The model under review builds one solid part; all positions refer to its coordinate system, in mm. A direction names the side the tool comes from. Coordinates: 2 decimals unless noted, no trailing zeros. Loops run counter-clockwise (first coordinate to the right, second up) from the corner with the lowest first, then second, coordinate; pieces in that order, holes last. Notation, with made-up numbers: M 17.5,80.5 L 45.5,80.5 A21 cw 45.5,86.5 Z; hole C -15,19 d2. An arc over 180 degrees is marked long. One line per item, written item: value.
```python
from build123d import *

# Parameters (mm, degrees)
SKETCH1_R               = 41.275
BOSS_EXTRUDE1_DEPTH     = 6.35
CUT_EXTRUDE1_DEPTH      = 60.737268518
CUT_EXTRUDE1_DEPTH_BACK = 60.737268518
SKETCH2_R               = 12.500000019
SKETCH3_R               = 16.000000004
CUT_EXTRUDE2_DEPTH      = 5


with BuildPart() as part:
    # Sketch1 → Boss-Extrude1 (new, symmetric)
    with BuildSketch(Plane.XY):
        Circle(SKETCH1_R)
    extrude(amount=BOSS_EXTRUDE1_DEPTH, both=True)

    # Sketch2 → Cut-Extrude1 (cut, two sides: drawn at the far end of the back side and taken through both)
    with BuildSketch(Plane.XY.offset(6.35).offset(-CUT_EXTRUDE1_DEPTH_BACK)):
        Circle(SKETCH2_R)
    extrude(amount=CUT_EXTRUDE1_DEPTH + CUT_EXTRUDE1_DEPTH_BACK, mode=Mode.SUBTRACT)

    # Sketch3 → Cut-Extrude2 (cut)
    with BuildSketch(Plane.XY.offset(6.35)):
        Circle(SKETCH3_R)
    extrude(amount=-CUT_EXTRUDE2_DEPTH, mode=Mode.SUBTRACT)


solid = part.part
```
(1) Add section A-A on x = 0. State the section outline as (y, z) points (3 decimals).
Checks:
outline: M -41.275,-6.35 L -12.5,-6.35 L -12.5,1.35 L -16,1.35 L -16,6.35 L -41.275,6.35 Z; M 12.5,-6.35 L 41.275,-6.35 L 41.275,6.35 L 16,6.35 L 16,1.35 L 12.5,1.35 Z
(2) Insertion check: pin 1 Ø1.5 at (y, z) = (12.5, -1.5) entering from +X; pin 2 Ø3 at (y, z) = (-20, 3) entering from +X; pin 3 Ø6 at (y, z) = (-27, -1) entering from +X. Each pin has a flat end and moves straight along its axis. Give the tip position at first contact, or say it passes through.
Checks:
pin 1: x = 39.57
pin 2: x = 36.9
pin 3: x = 33.58
(3) Add section C-C on z = -2.25. State the section outline as (x, y) points (3 decimals), then the cut area to 3 significant figures.
Checks:
outline: C 0,0 d82.55; hole C 0,0 d25
area: 4,860 mm^2
(4) To check wall thickness, follow L1, parallel to Y at x = 0, z = 3.95 (3 decimals); L2, parallel to Y at x = 0, z = -3.25 (3 decimals); L3, parallel to Y at x = -19, z = 1. State the ranges of each line that lie inside material, in increasing order. Write a range as [from, to].
Checks:
L1: [-41.275, -16], [16, 41.275]
L2: [-41.275, -12.5], [12.5, 41.275]
L3: [-36.64, 36.64]
(5) Draft analysis for pull direction Y (two halves, no side actions). For faces 3 (the face through (-8.948, -40.293, 0.089)), 4 (the face through (11.923, 3.755, -2.554)), 5 (the face through (-10, -9, -6.35)), state which applies: pulls with the +Y half, pulls with the -Y half, needs draft (parallel to the pull), parting line crosses it, or undercut.
Checks:
face 3: parting line crosses it
face 4: undercut
face 5: needs draft
(6) Add section D-D on y = 24. State the section outline as (x, z) points.
Checks:
outline: M -33.58,-6.35 L 33.58,-6.35 L 33.58,6.35 L -33.58,6.35 Z
(7) Tool access review of faces 1 (the face through (-10, -8, 1.35)), 2 (the face through (-1, -18, 6.35)): name each direction out of +Z, -Z, +X, -X, +Y, -Y from which nothing blocks a thin tool from reaching the whole face with its end or side.
Checks:
face 1: +Z
face 2: +Z, +X, -X, +Y, -Y
